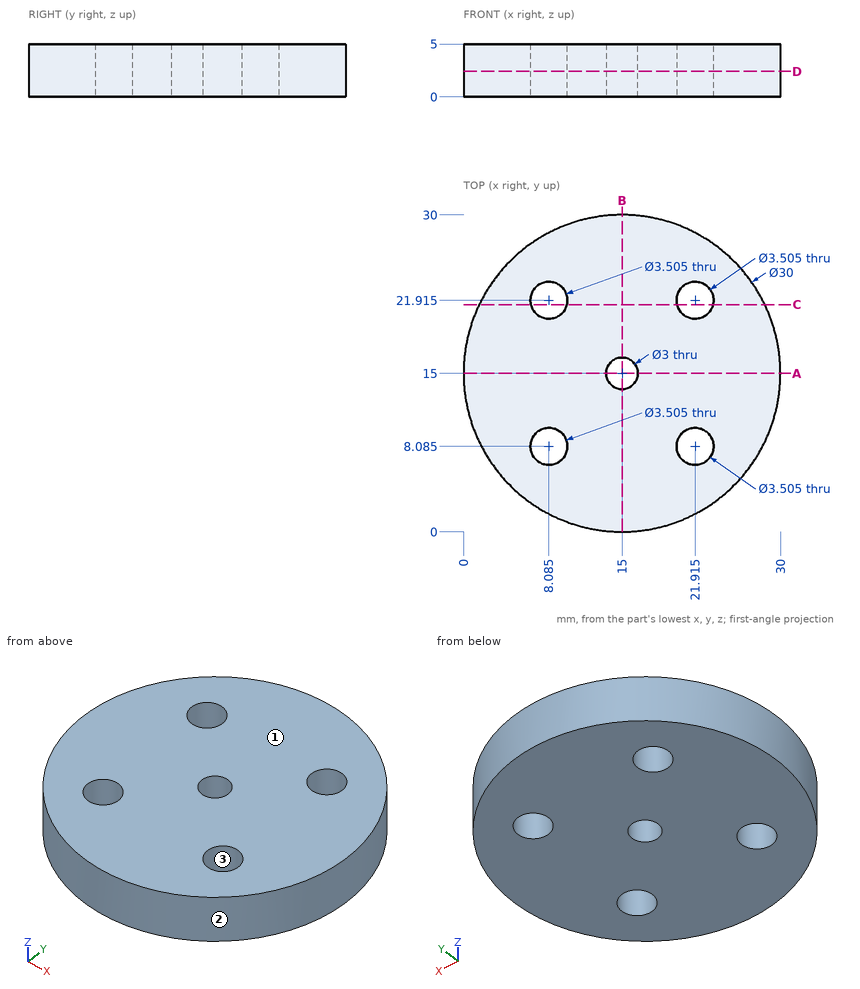
The drawing under review shows one solid part. Ordinate dimensions are in mm from its lowest x, y, z. Give positions to 0.01 mm unless a question says otherwise; leave off trailing zeros. Order: outer loops, then holes, each group sorted by start corner. A loop starts at its lowest first (then second) coordinate and runs counter-clockwise, first axis right, second up. Notation, with made-up numbers: M 70.25,43.25 L 97.25,43.25 A6 ccw 97.25,48.25 Z; hole C -11.5,-19 d4. An arc over 180 degrees is marked long. One line per question, with ' | ' between items. Start each with the question number.
Q1. The part is to be moulded in two halves that separate along X. For the marked faces 1, 2 and 3, say which applies: +X half, -X half, draft (parallel to the pull), parting line (faces both ways), or undercut.
Q2. We need section C-C (y = 21.5). Write out the cut boundary in (x, z), plus the area to 3 significant figures.
Q3. For L1, parallel to X at y = 8.5, z = 4.7; L2, parallel to Y at x = 7.5, z = 0.65; L3, parallel to X at y = 6.5, z = 1.35, list the stretches that pass through material, from the lowest coordinate up. Write a range as [from, to].
Q4. We need section A-A (y = 15). Write out the cut boundary in (x, z).
Q5. For pin 1 Ø2 at (x, z) = (8, 4.5) entering from +Y; pin 2 Ø1.5 at (y, z) = (12, 1.5) entering from +X, all flat-tipped, find the tip position at first contact; note any pin that passes through.
Q6. We need section D-D (z = 2.4). Write out the cut boundary in (x, y) (1 decimal).
Returned:
1) face 1: draft | face 2: parting line | face 3: undercut
2) outline: M 1.48,0 L 6.38,0 L 6.38,5 L 1.48,5 Z; M 9.79,0 L 20.21,0 L 20.21,5 L 9.79,5 Z; M 23.62,0 L 28.52,0 L 28.52,5 L 23.62,5 Z | area: 101 mm2
3) L1: [1.48, 6.38], [9.79, 20.21], [23.62, 28.52] | L2: [2.01, 6.43], [9.74, 20.26], [23.57, 27.99] | L3: [2.64, 7.34], [8.83, 21.17], [22.66, 27.36]
4) outline: M 0,0 L 13.5,0 L 13.5,5 L 0,5 Z; M 16.5,0 L 30,0 L 30,5 L 16.5,5 Z
5) pin 1: y = 28.75 | pin 2: x = 29.83
6) outline: C 15,15 d30; hole C 8.1,8.1 d3.5; hole C 8.1,21.9 d3.5; hole C 15,15 d3; hole C 21.9,8.1 d3.5; hole C 21.9,21.9 d3.5
